Can you work these out from the model? Positions are in its coordinate system, mm. A direction names the side the tool comes from. Give positions to 0.01 mm unless a question says otherwise; leave off trailing zeros. Order: outer loops, then holes, each group sorted by start corner. A loop starts at its lowest first (then second) coordinate and runs counter-clockwise, first axis right, second up.
```python
from build123d import *

# Parameters (mm, degrees)
F1_DEPTH       = 25
F2_R           = 5
F4_DEPTH       = 5.001
F6_D           = 4
F6_CBORE_D     = 8
F6_CBORE_DEPTH = 4


# Not quite as in the source:
# - a feature names something its author has since deleted; it is built from what else it names


with BuildPart() as f1:
    # F0 (on Top) → F1 (new body)
    with BuildSketch(Plane.XY):
        Polygon((0, 0), (0, -23), (5, -23), (5, -6), (40, -6), (40, 0), align=None)
    extrude(amount=F1_DEPTH)

    # F2
    f2_edges = [f1.edges().sort_by_distance(p)[0] for p in [
        (2.5, -23, 0),
        (2.5, -23, 25),
    ]]
    fillet(f2_edges, radius=F2_R)

    # F3 (on face) → F4 (cut, through all)
    with BuildSketch(Plane.YZ.offset(5)):
        with BuildLine():
            ThreePointArc((-17, 15), (-19, 13), (-17, 11))
            Line((-17, 11), (-10, 11))
            ThreePointArc((-10, 11), (-8, 13), (-10, 15))
            Line((-10, 15), (-17, 15))
        make_face()
    extrude(amount=-F4_DEPTH, mode=Mode.SUBTRACT)

    # F6 (through all)
    with Locations(Plane.XZ.offset(6)):
        with Locations((30, 12.5), (15, 12.5)):
            CounterBoreHole(F6_D / 2, F6_CBORE_D / 2, F6_CBORE_DEPTH)


solid = f1.part
```
1) I'm going to push flat-ended pins straight in: pin 1 Ø10 at (x, y) = (11, -18) entering from +Z; pin 2 Ø5 at (y, z) = (-10.5, 15) entering from +X; pin 3 Ø5 at (x, z) = (15, 12.5) entering from -Y; pin 4 Ø6.5 at (x, z) = (29, 14) entering from -Y. Where does each tip first touch, or does it pass through?
2) If I drill on line 1 (Z direction, x = 15, y = -5); line 2 (X direction, y = -4, z = 9.25); line 3 (Y direction, x = 37.5, z = 2.5), over which ranges is the centre line in solid material (lowest first)?
3) We'd pull the mould along Z, two halves only. Please class faces 1 (the face through (2, -23, 12)), 2 (the face through (17, -2, 11)), 3 (the face through (3, -22, 23)), 4 (the face through (3, -8, 13)): +Z half, -Z half, draft (parallel to the pull), parting line (faces both ways), or undercut.
4) Suppose I cut it at D-D (z = 13). Please give me the cut outline in (x, y), and give its area (3 significant figures).
5) Suppose I cut it at B-B (x = 15). Please give me the cut outline in (y, z), and give its area (3 significant figures).
6) Which directions (+Z, -Z, +X, -X, +Y, -Y) give clear straight access to the entire face, cutting with the end or side of a thin tool? Please do faces 5 (the face through (5, -15, 10)), 6 (the face through (27.05, -4.03, 15.2)), 7 (the face through (3, -14, 11)).
7) Suppose I cut it at A-A (y = -12.75). Please give me the cut outline in (x, z), and give its area (3 significant figures).
8) Suppose I cut it at C-C (z = 7.75). Please give me the cut outline in (x, y).
Results:
1. pin 1: passes through
1. pin 2: stops at x = 5
1. pin 3: stops at y = -2
1. pin 4: stops at y = -6
2. line 1: z = 0 to 8.5, 16.5 to 25
2. line 2: x = 0 to 12.67, 17.33 to 27.67, 32.33 to 40
2. line 3: y = -6 to 0
3. face 1: draft
3. face 2: undercut
3. face 3: +Z half
3. face 4: undercut
4. outline: (0, -23) - (5, -23) - (5, -19) - (0, -19) - close; (0, -8) - (5, -8) - (5, -6) - (11.03, -6) - (11.03, -2) - (13.06, -2) - (13.06, 0) - (0, 0) - close; (16.94, -2) - (18.97, -2) - (18.97, -6) - (26.03, -6) - (26.03, -2) - (28.06, -2) - (28.06, 0) - (16.94, 0) - close; (31.94, -2) - (33.97, -2) - (33.97, -6) - (40, -6) - (40, 0) - (31.94, 0) - close
4. area: 191 mm2
5. outline: (-6, 0) - (0, 0) - (0, 10.5) - (-2, 10.5) - (-2, 8.5) - (-6, 8.5) - close; (-6, 16.5) - (-2, 16.5) - (-2, 14.5) - (0, 14.5) - (0, 25) - (-6, 25) - close
5. area: 110 mm2
6. face 5: +Z, -Z, +X, -Y
6. face 6: -Y
6. face 7: +X, -X
7. outline: (0, 0) - (5, 0) - (5, 11) - (0, 11) - close; (0, 15) - (5, 15) - (5, 25) - (0, 25) - close
7. area: 105 mm2
8. outline: (0, -23) - (5, -23) - (5, -6) - (40, -6) - (40, 0) - (0, 0) - close
